Can you work these out from the drawing? Everything is in mm from the part's minimum corner. A direction names the side the tool comes from. Round coordinates to 2 decimals unless told otherwise and drop trailing zeros. Loops run counter-clockwise (first coordinate to the right, second up) from the corner with the lowest first, then second, coordinate; pieces in that order, holes last. Notation, with made-up numbers: (-25.75, 14) -> (8.25, 14) arc R16 ccw to (8.25, 26) -> close; hole circle Ø1 at (72.5, 16). An arc over 180 degrees is marked (long way). Answer as a JSON object with one key per item and string values.
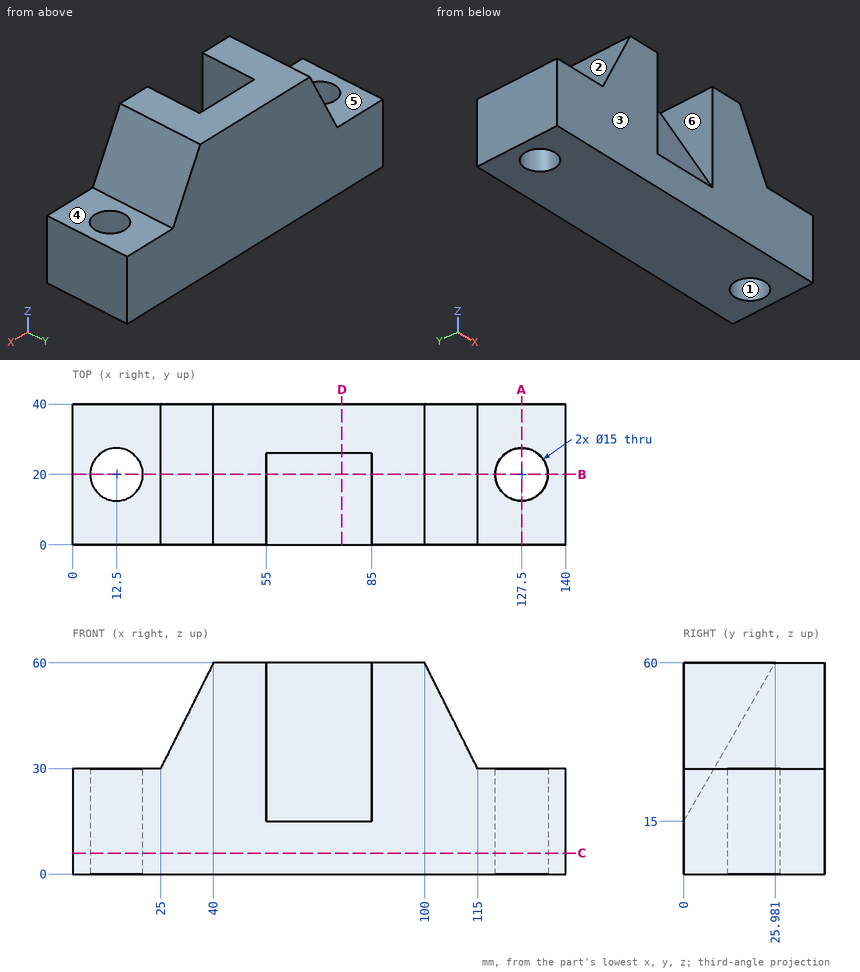
Q1. I want a section at C-C, the plane z = 6. Write out the boundary of the cut face in (x, y), then the cut area to 3 significant figures.
Determined:
{"outline": "(0, 0) -> (140, 0) -> (140, 40) -> (0, 40) -> close; hole circle Ø15 at (12.5, 20); hole circle Ø15 at (127.5, 20)", "area": "5,250 mm²"}
Q2. We'd pull the mould along X, two halves only. Please class the marked faces 1, 2 and 3: pulls with the +X half, pulls with the -X half, needs draft (parallel to the pull), parting line crosses it, or undercut.
Determined:
{"face 1": "undercut", "face 2": "pulls with the -X half", "face 3": "needs draft"}
Q3. I want a section at D-D, the plane x = 76.5. Write out the boundary of the cut face in (y, z), then the cut area to 3 significant figures.
Determined:
{"outline": "(0, 0) -> (40, 0) -> (40, 60) -> (25.98, 60) -> (0, 15) -> close", "area": "1,820 mm²"}
Q4. On a 3-axis mill with a long thin cutter (end or side, diameter ignored), from which of +Z, -Z, +X, -X, +Y, -Y can I reach the whole of each face in a straight line? I mean the marked faces 4, 5 and 6. Say none if no direction works.
Determined:
{"face 4": "+Z, +X, +Y, -Y", "face 5": "+Z, -X, +Y, -Y", "face 6": "+Z, -Y"}
Q5. I want a section at A-A, the plane x = 127.5. Write out the boundary of the cut face in (y, z).
Determined:
{"outline": "(0, 0) -> (12.5, 0) -> (12.5, 30) -> (0, 30) -> close; (27.5, 0) -> (40, 0) -> (40, 30) -> (27.5, 30) -> close"}
Q6. I want a section at B-B, the plane y = 20. Write out the boundary of the cut face in (x, z), then the cut area to 3 significant figures.
Determined:
{"outline": "(0, 0) -> (5, 0) -> (5, 30) -> (0, 30) -> close; (20, 0) -> (120, 0) -> (120, 30) -> (115, 30) -> (100, 60) -> (85, 60) -> (85, 49.64) -> (55, 49.64) -> (55, 60) -> (40, 60) -> (25, 30) -> (20, 30) -> close; (135, 0) -> (140, 0) -> (140, 30) -> (135, 30) -> close", "area": "5,240 mm²"}
Q7. If I drill on L1, parallel to X at y = 20, z = 10; L2, parallel to Y at x = 12.5, z = 10; L3, parallel to Y at x = 133, z = 26.5, over which ranges is the centre line in solid material (lowest first)? Write a range as [from, to].
Determined:
{"L1": "[0, 5], [20, 120], [135, 140]", "L2": "[0, 12.5], [27.5, 40]", "L3": "[0, 14.9], [25.1, 40]"}
Q8. I'm going to push flat-ended pins straight in: pin 1 (5 mm diameter, centred on y = 19.5, z = 46.5, fed in from +X); pin 2 (5 mm diameter, centred on y = 24.5, z = 35, fed in from -X); pin 3 (20 mm diameter, centred on x = 8.5, y = 24.5, fed in from +Z). Where does each tip first touch, or does it pass through?
Determined:
{"pin 1": "x = 108", "pin 2": "x = 26.25", "pin 3": "z = 30"}
